```python
from build123d import *

# Parameters (mm, degrees)
F0_R     = 1.0795
F1_DEPTH = 66.802
F2_R     = 1.0795
F3_DEPTH = 0.508
F4_R     = 1.2446
F4_R_2   = 1.0795
F5_DEPTH = 0.635


# Not quite as in the source:
# - a fillet or chamfer that OpenCascade refuses, or shapes differently, is made with other operations: its cross-section is extruded or revolved along the edge and cut away or added
# - two fillets or chamfers of one size are made in one step
# - a feature of the source that left no trace in its solid (it failed there, or was rolled back) is left out
# - a pattern or mirror of a feature is missing from the dataset's text; its kind, count and spacing are read off the source's solid


with BuildPart() as f1:
    # F0 (on Front) → F1 (new body)
    with BuildSketch(Plane.XZ):
        with Locations((9.3034878373, 10.9315989539)):
            Circle(F0_R)
    extrude(amount=F1_DEPTH)

    # F2 (on face) → F3 (join)
    with BuildSketch(Plane(origin=(0, 0, 0), x_dir=(-1, 0, 0), z_dir=(0, 1, 0))):
        with Locations((-9.3034878373, 10.9315989539)):
            Circle(F2_R)
    extrude(amount=F3_DEPTH)

    # F4 (on face) → F5 (join)
    with BuildSketch(Plane.XZ.offset(66.802)):
        with Locations((9.3034878373, 10.9315989539)):
            Circle(F4_R)
        with Locations((9.3034878373, 10.9315989539)):
            Circle(F4_R_2, mode=Mode.SUBTRACT)
        with Locations((9.3034878373, 10.9315989539)):
            Circle(F4_R_2)
    f5 = extrude(amount=F5_DEPTH)

    # F5_copies: F5 across plane
    add(f5.mirror(Plane.ZX.offset(-33.147)))

    # F8: chamfer of 0.6858 on 2 edges, made by hand

    # F8_s1 → F8_t2 (revolve, cut)
    with BuildSketch(Plane.XY.offset(10.9315989539)):
        Polygon((10.5480878373, 0.4572), (9.8622878373, 1.143), (10.5480878373, 1.143), align=None)
    revolve(axis=Axis((9.3034878373, 1.143, 10.9315989539), (0, -1, 0)), mode=Mode.SUBTRACT)

    # F8_s3 → F8_t4 (revolve, cut)
    with BuildSketch(Plane.XY.offset(10.9315989539)):
        Polygon((10.5480878373, -66.7512), (9.8622878373, -67.437), (10.5480878373, -67.437), align=None)
    revolve(axis=Axis((9.3034878373, -67.437, 10.9315989539), (0, -1, 0)), mode=Mode.SUBTRACT)


solid = f1.part
```
The listing builds one solid part. Answer for the finished solid, in the listing's coordinates (mm). Give positions to 0.01 mm unless a question says otherwise; leave off trailing zeros. Loops run counter-clockwise (first coordinate to the right, second up) from the corner with the lowest first, then second, coordinate; pieces in that order, holes last. Notation, with made-up numbers: M -32.5,13.25 L 10.5,13.25 A22 cw 10.5,31.25 Z; hole C -26.5,47 d9. An arc over 180 degrees is marked long. One line per item, written item: value.
Q1. A cutting plane is placed at A-A on y = -32.5. Determine the outline of the cut face in (x, z).
Working result:
outline: C 9.3,10.93 d2.16
Q2. Find the intervals of material crossed by line 1 (Y direction, x = 9.1, z = 10.4); line 2 (Z direction, x = 9.4, y = -51); line 3 (X direction, y = -14, z = 11.1), in increasing order. Write a range as from..to.
Working result:
line 1: y = -67.43..1.13
line 2: z = 9.86..12.01
line 3: x = 8.24..10.37
Q3. A flat-ended cylindrical pin translates along its axis: P1, Ø1, axis at x = 8.5, z = 11.5, coming from the +Y side. Find the tip coordinate at first contact, or state that the pin passes through.
Working result:
P1: stops at y = 1.14
